Model file for the job. Use its own axes, mm. A direction names the side the tool comes from. Give positions to 0.01 mm unless a question says otherwise; leave off trailing zeros. Loops run counter-clockwise (first coordinate to the right, second up) from the corner with the lowest first, then second, coordinate; pieces in that order, holes last. Notation, with made-up numbers: M 33,35.25 L 57,35.25 A22 cw 57,52.25 Z; hole C -7,66.25 d4. An arc over 180 degrees is marked long. Answer in a Markdown table with one row per item.
Autodesk Inventor part; units mm, degrees
ref_plane "YZ Plane" through (0, 0, 0) normal (1, 0, 0) x (0, 1, 0)
ref_plane "XZ Plane" through (0, 0, 0) normal (0, 1, 0) x (-1, 0, 0)
ref_plane "XY Plane" through (0, 0, 0) normal (0, 0, 1) x (1, 0, 0)
sketch "Sketch1" plane through (0, 0, 0) normal (1, 0, 0) x (0, 1, 0)
  line L0 (0, 0) -> (25.4, 0)
  line L1 (25.4, 0) -> (25.4, -25.4)
  line L2 (25.4, -25.4) -> (0, -25.4)
  line L3 (0, -25.4) -> (0, 0)
  line L4 (23.8125, -23.8125) -> (23.8125, -1.5875)
  line L5 (23.8125, -1.5875) -> (1.5875, -1.5875)
  line L6 (1.5875, -1.5875) -> (1.5875, -23.8125)
  line L7 (1.5875, -23.8125) -> (23.8125, -23.8125)
  dimension "d0" = 25.4
  dimension "d1" = 25.4
  dimension "d2" = 1.5875
extrude "Extrusion1" add sketch "Sketch1" along normal mid plane 63.5
sketch "Sketch3" plane through (-31.75, 0, 0) normal (0, 0, 1) x (1, 0, 0)
  line L0 (0, 0) -> (63.5, 0)
  line L1 (63.5, 25.4) -> (63.5, 0)
  line L2 (0, 25.4) -> (63.5, 25.4)
  line L3 (0, 0) -> (0, 25.4)
  circle A0 centre (19.05, 12.7) radius 2.5781
  circle A1 centre (44.45, 12.7) radius 2.5781
  line L4 (31.75, 25.4) -> (31.75, 0) construction
  dimension "d14" = 5.1562
  dimension "d15" = 5.1562
  dimension "d16" = 12.7
  dimension "d17" = 25.4
  dimension "d20" = 12.7
extrude "Extrusion3" cut sketch "Sketch3" against normal blind 25.4 contours A0 | A1
properties part number "1inTubeBase"
(1) Saw through at C-C, the plane x = -23.5. Give the cut face in (y, z), and give its area (3 significant figures).
Established:
| item | result |
|---|---|
| outline | M 0,-25.4 L 25.4,-25.4 L 25.4,0 L 0,0 Z; hole M 1.59,-23.81 L 23.81,-23.81 L 23.81,-1.59 L 1.59,-1.59 Z |
| area | 151 mm2 |
(2) Which spindle directions (+Z, -Z, +X, -X, +Y, -Y) get a long thin tool onto all of the face, cutting with end or side? Do faces 1 (the flat face through (0, 13, -23.812)), 2 (the cylindrical face through (15.16, 13.47, -24.6)). Say none if no direction does.
Established:
| item | result |
|---|---|
| face 1 | +X, -X |
| face 2 | +Z, -Z |
(3) Flat gauge pin, fed straight in: P1, Ø2, axis at y = 21, z = -7.5, coming from the -X side. Where does the tip first touch, or does it go through?
Established:
| item | result |
|---|---|
| P1 | passes through |
(4) Saw through at A-A, the plane y = 12.7. Give the cut face in (x, z), and give its area (3 significant figures).
Established:
| item | result |
|---|---|
| outline | M -31.75,-25.4 L -15.28,-25.4 L -15.28,-23.81 L -31.75,-23.81 Z; M -31.75,-1.59 L -15.28,-1.59 L -15.28,0 L -31.75,0 Z; M -10.12,-25.4 L 10.12,-25.4 L 10.12,-23.81 L -10.12,-23.81 Z; M -10.12,-1.59 L 10.12,-1.59 L 10.12,0 L -10.12,0 Z; M 15.28,-25.4 L 31.75,-25.4 L 31.75,-23.81 L 15.28,-23.81 Z; M 15.28,-1.59 L 31.75,-1.59 L 31.75,0 L 15.28,0 Z |
| area | 169 mm2 |
(5) Saw through at D-D, the plane y = 9.5. Give the cut face in (x, z), and give its area (3 significant figures).
Established:
| item | result |
|---|---|
| outline | M -31.75,-25.4 L 31.75,-25.4 L 31.75,-23.81 L -31.75,-23.81 Z; M -31.75,-1.59 L 31.75,-1.59 L 31.75,0 L -31.75,0 Z |
| area | 202 mm2 |
(6) Mould opens along X. For faces 3 (the cylindrical face through (15.16, 13.47, -0.78)), 4 (the flat face through (-31.75, 1, -13)), 5 (the flat face through (0, 0, -13)) say: pulls with the +X half, pulls with the -X half, needs draft (parallel to the pull), parting line crosses it, or undercut.
Established:
| item | result |
|---|---|
| face 3 | undercut |
| face 4 | pulls with the -X half |
| face 5 | needs draft |
(7) Wall check: L1, parallel to Z at x = 5, y = 23.5; L2, parallel to Y at x = 12.7, z = -0.8; L3, parallel to Y at x = -13.5, z = -5.5. Give the ranges that are in metal, low to high.
Established:
| item | result |
|---|---|
| L1 | z = -25.4 to -23.81, -1.59 to 0 |
| L2 | y = 0 to 10.12, 15.28 to 25.4 |
| L3 | y = 0 to 1.59, 23.81 to 25.4 |
(8) Saw through at B-B, the plane z = -14.5. Give the cut face in (x, y), and give its area (3 significant figures).
Established:
| item | result |
|---|---|
| outline | M -31.75,0 L 31.75,0 L 31.75,1.59 L -31.75,1.59 Z; M -31.75,23.81 L 31.75,23.81 L 31.75,25.4 L -31.75,25.4 Z |
| area | 202 mm2 |
